Answer from the drawing. Dimensions are ordinates in mm from the lowest x, y and z of the part. A direction names the side the tool comes from. Give positions to 0.01 mm unless a question says otherwise; leave off trailing zeros. Loops run counter-clockwise (first coordinate to the right, second up) from the corner with the lowest first, then second, coordinate; pieces in that order, holes last. Notation, with made-up numbers: (81.25, 17.25) -> (99.25, 17.25) arc R21 cw to (99.25, 56.25) -> close; hole circle Ø4 at (83.25, 35.25). An arc over 180 degrees is marked (long way). Return JSON: item names as keys, results as strings. Group by question number.
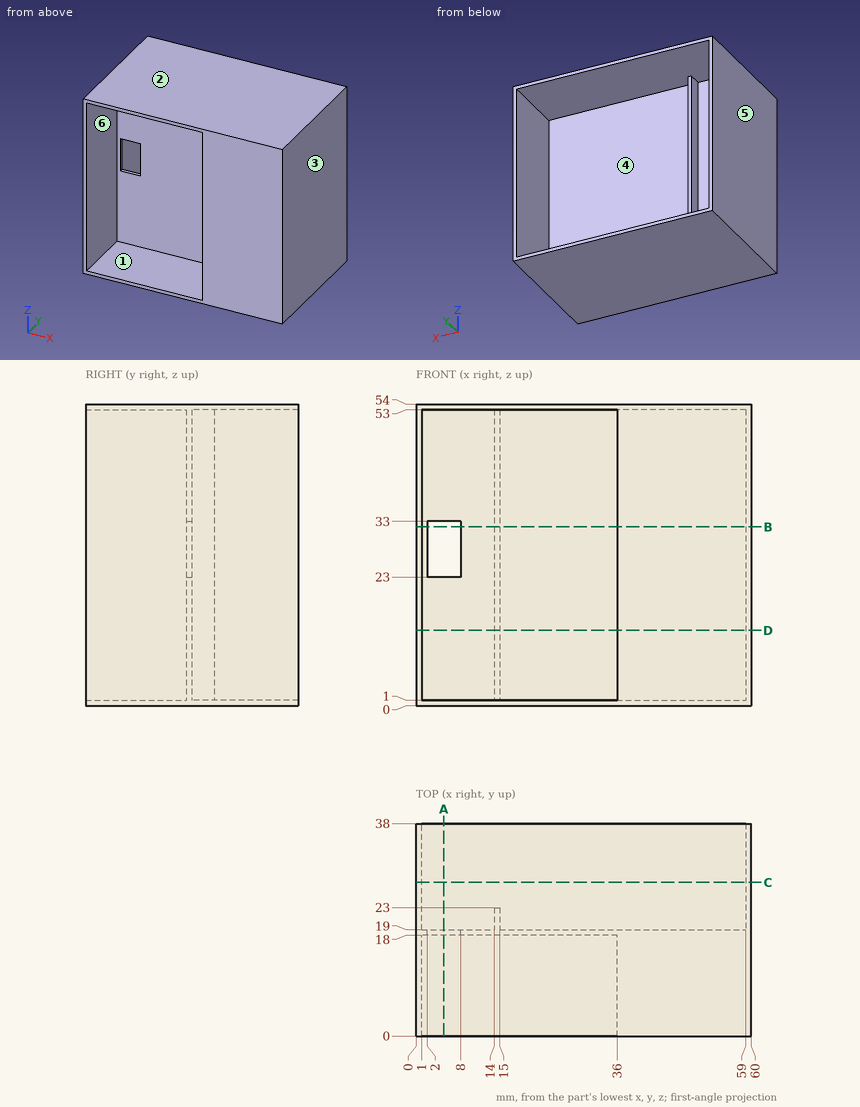
1. Flat-ended cylindrical pins translate along their axes: pin 1 Ø10.5 at (x, z) = (9, 34.5) entering from +Y; pin 2 Ø10.5 at (x, z) = (10, 17.5) entering from -Y; pin 3 Ø3 at (x, z) = (40.5, 8) entering from +Y. Find the tip coordinate at first contact, or state that the pin passes through.
2. Section D-D on z = 13.5 is taken. Determine the outline of the cut face in (x, y).
3. Straight lines are drawn through the part: line 1 (X direction, y = 14.5, z = 24.5); line 2 (Z direction, x = 14.5, y = 12); line 3 (X direction, y = 27, z = 42.5). For each, find the intervals that lie inside material, in ascending order. Write a range as from..to.
4. Determine the mould class of the marked faces 1, 2 and 3 for opening direction Z: pulls with the +Z half, pulls with the -Z half, needs draft (parallel to the pull), parting line crosses it, or undercut.
5. Section B-B on z = 32 is taken. Determine the outline of the cut face in (x, y).
6. Section C-C on y = 27.5 is taken. Determine the outline of the cut face in (x, z).
7. Section A-A on x = 5 is taken. Determine the outline of the cut face in (y, z).
8. Which of the six approach directions +Z, -Z, +X, -X, +Y, -Y give full straight-line access (tool end or side, diameter ignored) to the marked faces 4, 5 and 6?
Completed:
{
 "1": {"pin 1": "stops at y = 23", "pin 2": "stops at y = 18", "pin 3": "stops at y = 19"},
 "2": {"outline": "(0, 0) -> (1, 0) -> (1, 18) -> (36, 18) -> (36, 0) -> (60, 0) -> (60, 38) -> (59, 38) -> (59, 19) -> (15, 19) -> (15, 23) -> (14, 23) -> (14, 19) -> (1, 19) -> (1, 38) -> (0, 38) -> close"},
 "3": {"line 1": "x = 0..1, 36..60", "line 2": "z = 0..1, 53..54", "line 3": "x = 0..1, 59..60"},
 "4": {"face 1": "undercut", "face 2": "pulls with the +Z half", "face 3": "needs draft"},
 "5": {"outline": "(0, 0) -> (1, 0) -> (1, 18) -> (2, 18) -> (2, 19) -> (1, 19) -> (1, 38) -> (0, 38) -> close; (8, 18) -> (36, 18) -> (36, 0) -> (60, 0) -> (60, 38) -> (59, 38) -> (59, 19) -> (15, 19) -> (15, 23) -> (14, 23) -> (14, 19) -> (8, 19) -> close"},
 "6": {"outline": "(0, 0) -> (60, 0) -> (60, 54) -> (0, 54) -> close; hole (1, 1) -> (59, 1) -> (59, 53) -> (1, 53) -> close"},
 "7": {"outline": "(0, 0) -> (38, 0) -> (38, 1) -> (19, 1) -> (19, 23) -> (18, 23) -> (18, 1) -> (0, 1) -> close; (0, 53) -> (18, 53) -> (18, 33) -> (19, 33) -> (19, 53) -> (38, 53) -> (38, 54) -> (0, 54) -> close"},
 "8": {"face 4": "+Y", "face 5": "+Z, -Z, -X, +Y, -Y", "face 6": "-Y"}
}
